from build123d import *

# Parameters (mm, degrees)
F1_R     = 12.5
F2_DEPTH = 13
F0_R     = 22.5
F3_DEPTH = 10
F5_R     = 3
F6_SIZE  = 3
F8_DEPTH = 9


# Not quite as in the source:
# - the program builds the solid bodies; features that only make, move or delete a surface that nothing else refers to are left out


with BuildPart() as f2:
    # F1 (on Top) → F2 (new body)
    with BuildSketch(Plane.XY):
        with Locations((-37.169251591, 37.6385599375)):
            Circle(F1_R)
    extrude(amount=F2_DEPTH)

    # F3 (add): a face of the model
    f3_faces = [f2.faces().sort_by_distance(p)[0] for p in [
        (-37.169251591, 37.6385599375, 13),
    ]]


with BuildPart() as f2b:
    # F0 (on Top) → F2, piece 2 (new body)
    with BuildSketch(Plane.XY):
        with Locations((-37.3275603359, 37.7723030881)):
            Circle(F0_R)
    extrude(amount=F2_DEPTH)


with BuildPart() as f2_1:
    add(f2.part)

    add(f2b.part)  # F3 merges F2b
    extrude(f3_faces, amount=F3_DEPTH)

    # F5
    f5_edges = [f2_1.edges().sort_by_distance(p)[0] for p in [
        (-59.82756, 37.772303, 13),
        (-59.82756, 37.772303, 0),
    ]]
    fillet(f5_edges, radius=F5_R)

    # F6
    f6_edges = [f2_1.edges().sort_by_distance(p)[0] for p in [
        (-49.669252, 37.63856, 23),
    ]]
    chamfer(f6_edges, length=F6_SIZE)

    # F4 (on face) → F8 (cut)
    with BuildSketch(Plane.XY.offset(23)):
        Polygon((-36.4021524321, 30.1723097264), (-30.3197396578, 34.5697621907), (-31.0868388166, 42.0360124018), (-37.9363507498, 45.1048101485), (-44.0187635242, 40.7073576842), (-43.2516643653, 33.2411074732), align=None)
    extrude(amount=-F8_DEPTH, mode=Mode.SUBTRACT)


solid = f2_1.part
Source: CAD feature listing. Evaluate the final solid. Frame: model axes, mm. A direction names the side the tool comes from. Round coordinates to 2 decimals unless told otherwise and drop trailing zeros. Loops run counter-clockwise (first coordinate to the right, second up) from the corner with the lowest first, then second, coordinate; pieces in that order, holes last.
Q1. Mould query, pull axis Y, two halves, no side actions, for faces 3 (the face through (-38, 25, 13)), 4 (the face through (-33.404, 32.34, 18.563)), 5 (the face through (-31.984, 45.772, 22.854)). Classes: pulls with the +Y half, pulls with the -Y half, needs draft (parallel to the pull), parting line crosses it, or undercut.
Q2. Section A-A, the plane z = 18. Return loops of the section in (x, y).
Q3. Ray query, line 1 (Z direction, x = -38, y = 18); line 2 (X direction, y = 38, z = 7); line 3 (Z direction, x = -35, y = 40.5). Return the intervals inside material, ascending.
Q4. First-contact query: P1, Ø6, axis at y = 24.5, z = 9.5, coming from the +X side; P2, Ø1, axis at y = 28, z = 14, coming from the -X side; P3, Ø6, axis at x = -50.5, z = 20.5, coming from the +Y side; P4, Ø1.5, axis at x = -19.5, y = 22.5, coming from the -Z side. Flat tips, straight axial feed; report the tip coordinate or a pass-through.
Q5. Section B-B, the plane z = 2. Return loops of the section in (x, y).
Q6. Access query for faces 1 (the face through (-39, 31, 23)), 2 (the face through (-37, 38, 14)). Directions: +Z, -Z, +X, -X, +Y, -Y. A direction counts if a zero-diameter tool reaches every point of the face in a straight line with its end or side. Return the directions, or none.
Solutions:
1. face 3: needs draft
1. face 4: undercut
1. face 5: parting line crosses it
2. outline: circle Ø25 at (-37.17, 37.64); hole (-44.02, 40.71) - (-43.25, 33.24) - (-36.4, 30.17) - (-30.32, 34.57) - (-31.09, 42.04) - (-37.94, 45.1) - close
3. line 1: z = 0.01 to 12.99
3. line 2: x = -59.83 to -14.83
3. line 3: z = 0 to 14
4. P1: stops at x = -17.31
4. P2: stops at x = -45.7
4. P3: stops at y = 44.61
4. P4: passes through
5. outline: circle Ø44.66 at (-37.33, 37.77)
6. face 1: +Z, +X, -X, +Y, -Y
6. face 2: +Z
